Check sheet for the modelled part. Datum: model origin and axes. Units: mm. A direction names the side the tool comes from. Round coordinates to 2 decimals unless told otherwise and drop trailing zeros. Write each loop counter-clockwise with the first axis right and the second up, starting at its lowest first coordinate (ties: lowest second). Pieces come first, ordered by that corner, then holes. Notation, with made-up numbers: (-38.5, -6.5) - (1.5, -6.5) arc R26 cw to (1.5, 22.5) - close; hole circle Ø3 at (-6, 34.5). An arc over 180 degrees is marked (long way). Answer as a JSON object with one key per item and string values. Group by question number.
Item 1: Thickness scan on line 1 (Y direction, x = 23, z = 234); line 2 (X direction, y = 107, z = 235); line 3 (Z direction, x = 361, y = 57). Record the ranges inside material, lowest first.
Item 2: Set-up check for faces 4 (the flat face through (198, 77, 25.4)), 5 (the flat face through (401.32, 75, 259)): record each of +Z, -Z, +X, -X, +Y, -Y from which the full face is reachable in a straight line by a thin tool's end or side.
Item 3: Sectioned sample at B-B on y = 17. Record the boundary of the cut face in (x, z), plus the area to 3 significant figures.
Item 4: Gauge pin test, flat end, axial feed: P1, Ø1.5, axis at x = 168.5, y = 49, coming from the -Z side. Record the tip position at first contact, or that the pin passes through.
Item 5: Sectioned sample at A-A on z = 355. Record the boundary of the cut face in (x, y), plus the area to 3 significant figures.
Item 6: Sectioned sample at C-C on x = 313.5. Count the separate pieces of the cut face and the enclosed holes in it, plus the area to 3 significant figures.
Item 7: Release check for a two-part mould opening along Z. For faces 1 (the flat face through (198, 0, 259)), 2 (the flat face through (198, 77, 0)), 3 (the flat face through (398.78, 77, 278)) record: pulls with the +Z half, pulls with the -Z half, needs draft (parallel to the pull), parting line crosses it, or undercut.
```python
from build123d import *

# Parameters (mm, degrees)
SKETCH2_W           = 401.32
SKETCH2_H           = 152.4
BOSS_EXTRUDE1_DEPTH = 525.78
SKETCH3_W           = 396.24
SKETCH3_H           = 497.84
CUT_EXTRUDE1_DEPTH  = 149.86
SKETCH4_W           = 396.24
SKETCH4_H           = 497.84
BOSS_EXTRUDE3_DEPTH = 2.54
SKETCH8_W           = 254
SKETCH8_H           = 12.7
CUT_EXTRUDE2_DEPTH  = 2.54
CUT_EXTRUDE2_TAPER  = 15


with BuildPart() as part:
    # Sketch2 → Boss-Extrude1 (new body)
    with BuildSketch(Plane.XY):
        with Locations((200.66, 76.2)):
            Rectangle(SKETCH2_W, SKETCH2_H)
    extrude(amount=BOSS_EXTRUDE1_DEPTH)

    # Sketch3 → Cut-Extrude1 (cut)
    with BuildSketch(Plane(origin=(0, 152.4, 0), x_dir=(1, 0, 0), z_dir=(0, 1, 0))):
        with Locations((200.66, -274.32)):
            Rectangle(SKETCH3_W, SKETCH3_H)
    extrude(amount=-CUT_EXTRUDE1_DEPTH, mode=Mode.SUBTRACT)

    # Sketch4 → Boss-Extrude3 (add)
    with BuildSketch(Plane(origin=(0, 152.4, 0), x_dir=(1, 0, 0), z_dir=(0, 1, 0))):
        with Locations((200.66, -274.32)):
            Rectangle(SKETCH4_W, SKETCH4_H)
    extrude(amount=-BOSS_EXTRUDE3_DEPTH)

    # Sketch8 → Cut-Extrude2 (cut)
    with BuildSketch(Plane(origin=(0, 152.4, 0), x_dir=(1, 0, 0), z_dir=(0, 1, 0))):
        with Locations((200.66, -273.05)):
            Rectangle(SKETCH8_W, SKETCH8_H)
        with Locations((200.66, -234.95)):
            Rectangle(SKETCH8_W, SKETCH8_H)
        with Locations((200.66, -311.15)):
            Rectangle(SKETCH8_W, SKETCH8_H)
    extrude(amount=-CUT_EXTRUDE2_DEPTH, taper=CUT_EXTRUDE2_TAPER, mode=Mode.SUBTRACT)


solid = part.part
```
Completed:
{
 "1": {"line 1": "0 to 2.54, 149.86 to 152.4", "line 2": "0 to 2.54, 398.78 to 401.32", "line 3": "0 to 25.4, 523.24 to 525.78"},
 "2": {"face 4": "none", "face 5": "+Z, -Z, +X, +Y, -Y"},
 "3": {"outline": "(0, 0) - (401.32, 0) - (401.32, 525.78) - (0, 525.78) - close; hole (2.54, 25.4) - (398.78, 25.4) - (398.78, 523.24) - (2.54, 523.24) - close", "area": "13,700 mm²"},
 "4": {"P1": "z = 0"},
 "5": {"outline": "(0, 0) - (401.32, 0) - (401.32, 152.4) - (0, 152.4) - close; hole (2.54, 2.54) - (398.78, 2.54) - (398.78, 149.86) - (2.54, 149.86) - close", "area": "2,790 mm²"},
 "6": {"separate pieces": "3", "enclosed holes": "0", "area": "6,700 mm²"},
 "7": {"face 1": "needs draft", "face 2": "pulls with the -Z half", "face 3": "undercut"}
}
